```python
from build123d import *

# Parameters (mm, degrees)
SKETCH_1_W             = 5
SKETCH_1_H             = 3.7
EXTRUDE_1_DEPTH        = 37.5
SKETCH_2_R             = 1.2
CUT_EXTRUDE_1_DEPTH    = 3010.5
SKETCH_3_R             = 1.8
CUT_EXTRUDE_2_DEPTH    = 0.8
PATTERN_LINEAR_1_COUNT = 5
PATTERN_LINEAR_1_PITCH = 15


with BuildPart() as part:
    # 草图1 → 凸台-拉伸1 (new, symmetric)
    with BuildSketch(Plane.XY):
        Rectangle(SKETCH_1_W, SKETCH_1_H)
    extrude(amount=EXTRUDE_1_DEPTH, both=True)

    # 草图2 → 切除-拉伸1 (cut, symmetric)
    with BuildSketch(Plane(origin=(0, 1.85, 0), x_dir=(1, 0, 0), z_dir=(0, 1, 0))):
        with Locations(Location((0, -30, 0), (0, 0, 270))):
            Circle(SKETCH_2_R)
    cut_extrude_1 = extrude(amount=CUT_EXTRUDE_1_DEPTH, both=True, mode=Mode.SUBTRACT)

    # 草图3 → 切除-拉伸2 (cut)
    with BuildSketch(Plane(origin=(0, 1.85, 0), x_dir=(1, 0, 0), z_dir=(0, 1, 0))):
        with Locations(Location((0, -30, 0), (0, 0, 270))):
            Circle(SKETCH_3_R)
    cut_extrude_2 = extrude(amount=-CUT_EXTRUDE_2_DEPTH, mode=Mode.SUBTRACT)

    # 阵列(线性)1: 切除-拉伸1, 切除-拉伸2 ×5
    with Locations(*[(0, 0, -i * PATTERN_LINEAR_1_PITCH) for i in range(1, PATTERN_LINEAR_1_COUNT)]):
        add(cut_extrude_1, mode=Mode.SUBTRACT)
        add(cut_extrude_2, mode=Mode.SUBTRACT)


solid = part.part
```
Build history of the part. All positions in model axes, mm. A direction names the side the tool comes from. Round coordinates to 2 decimals unless told otherwise and drop trailing zeros. Write each loop counter-clockwise with the first axis right and the second up, starting at its lowest first coordinate (ties: lowest second). Pieces come first, ordered by that corner, then holes. Notation, with made-up numbers: (-6, 39.5) -> (50, 39.5) arc R6 ccw to (50, 44.5) -> close; hole circle Ø7 at (82, 46). An arc over 180 degrees is marked (long way). Put each result on its own line as item: value.
Item 1: Wall check: probe 1 along Z at (x, y) = (0.2, 0.5); probe 2 along Z at (x, y) = (-0.35, 1.3); probe 3 along X at (y, z) = (1.35, 30). Give the ranges that are in metal, low to high. Write a range as from..to.
Here are the results:
probe 1: z = -37.5..-31.18, -28.82..-16.18, -13.82..-1.18, 1.18..13.82, 16.18..28.82, 31.18..37.5
probe 2: z = -37.5..-31.77, -28.23..-16.77, -13.23..-1.77, 1.77..13.23, 16.77..28.23, 31.77..37.5
probe 3: x = -2.5..-1.8, 1.8..2.5
Item 2: Flat gauge pins, fed straight in: P1, Ø3, axis at x = 0, z = -15, coming from the +Y side; P2, Ø3, axis at x = -0.5, z = 0.5, coming from the +Y side. Where does each tip first touch, or does it go through?
Here are the results:
P1: stops at y = 1.05
P2: stops at y = 1.85
Item 3: Slice it at C-C, the plane x = 0. Count the separate pieces of the cut face and the enclosed holes in it, plus the area to 3 significant figures.
Here are the results:
separate pieces: 6
enclosed holes: 0
area: 228 mm^2
Item 4: Slice it at B-B, the plane y = -0.35. Give the cut face in (x, z), plus the area to 3 significant figures.
Here are the results:
outline: (-2.5, -37.5) -> (2.5, -37.5) -> (2.5, 37.5) -> (-2.5, 37.5) -> close; hole circle Ø2.4 at (0, -30); hole circle Ø2.4 at (0, -15); hole circle Ø2.4 at (0, 0); hole circle Ø2.4 at (0, 15); hole circle Ø2.4 at (0, 30)
area: 352 mm^2
Item 5: Slice it at A-A, the plane z = -15. Give the cut face in (x, y).
Here are the results:
outline: (-2.5, -1.85) -> (-1.2, -1.85) -> (-1.2, 1.05) -> (-1.8, 1.05) -> (-1.8, 1.85) -> (-2.5, 1.85) -> close; (1.2, -1.85) -> (2.5, -1.85) -> (2.5, 1.85) -> (1.8, 1.85) -> (1.8, 1.05) -> (1.2, 1.05) -> close
Item 6: Two-plate mould, pull along Z, no slides. Class faces 1 (the face through (-1, -1.85, 1)), 2 (the face through (0.541, 1.456, -13.283)), 3 (the face through (0, 0, 37.5)): pulls with the +Z half, pulls with the -Z half, needs draft (parallel to the pull), parting line crosses it, or undercut.
Here are the results:
face 1: needs draft
face 2: undercut
face 3: pulls with the +Z half
Item 7: Tool access for faces 4 (the face through (0.541, 1.456, 16.717)), 5 (the face through (-2.5, 0, 1)): list every direction of +Z, -Z, +X, -X, +Y, -Y with a clear straight run to the whole face (end or side of a thin tool).
Here are the results:
face 4: +Y
face 5: +Z, -Z, -X, +Y, -Y
